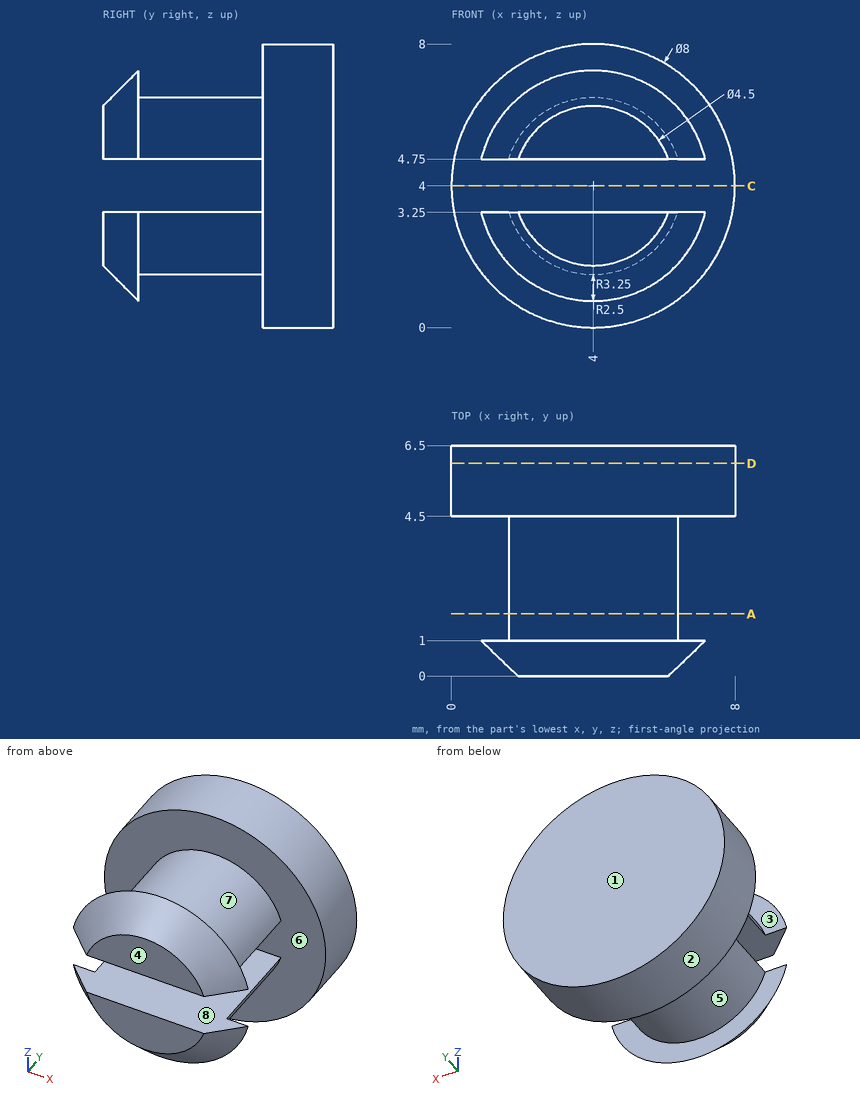
Print and shaded views of the part. All mm, measured from the part's lowest x, y and z. A direction names the side the tool comes from. Round coordinates to 2 decimals unless told otherwise and drop trailing zeros. Loops run counter-clockwise (first coordinate to the right, second up) from the corner with the lowest first, then second, coordinate; pieces in that order, holes last. Notation, with made-up numbers: M 72.5,-18.5 L 126.5,-18.5 A19 cw 126.5,4.5 Z; hole C -13.5,79.25 d11. An arc over 180 degrees is marked long. One line per question, with ' | ' between items.
1) Band-saw the part on D-D (y = 6). Give the cut face in (x, z).
Solved:
outline: C 4,4 d8
2) Flat gauge pins, fed straight in: pin 1 (1 mm diameter, centred on x = 3, y = 3, fed in from +Z); pin 2 (1.5 mm diameter, centred on y = 2.5, z = 5, fed in from -X); pin 3 (2 mm diameter, centred on x = 2.5, y = 2.5, fed in from -Z). Where does each tip first touch, or does it go through?
Solved:
pin 1: stops at z = 6.45 | pin 2: stops at x = 1.62 | pin 3: stops at z = 1.55
3) Drill centre lines: line 1 along Y through (x, z) = (6, 7); line 2 along Z through (x, y) = (3, 1.5); line 3 along Y through (x, z) = (6.5, 5.5). Where is each one in solid material? Low to high.
Solved:
line 1: y = 4.5 to 6.5 | line 2: z = 1.71 to 3.25, 4.75 to 6.29 | line 3: y = 0.67 to 1, 4.5 to 6.5
4) 3-axis set-ups, long thin cutter, end or side, ignore diameter. For the marked faces 5, 6, 7 and 8: which of +Z, -Z, +X, -X, +Y, -Y reach the whole face in a straight line?
Solved:
face 5: -Z | face 6: none | face 7: +Z | face 8: +X, -X, -Y
5) Band-saw the part on C-C (z = 4). Give the cut face in (x, y).
Solved:
outline: M 0,4.5 L 8,4.5 L 8,6.5 L 0,6.5 Z
6) Band-saw the part on A-A (y = 1.75). Give the cut face in (x, z), then the cut area to 3 significant figures.
Solved:
outline: M 1.62,3.25 A2.5 ccw 6.38,3.25 Z; M 1.62,4.75 L 6.38,4.75 A2.5 ccw Z | area: 12.2 mm²
7) Mould opens along Y. For the marked faces 1, 2, 3 and 4 say: +Y half, -Y half, draft (parallel to the pull), parting line (faces both ways), or undercut.
Solved:
face 1: +Y half | face 2: draft | face 3: undercut | face 4: -Y half
